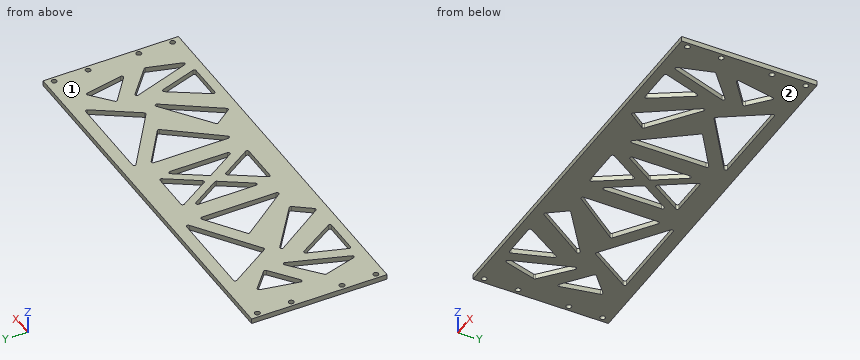
from build123d import *

# Parameters (mm, degrees)
SKETCH_1_W             = 230
SKETCH_1_H             = 80
EXTRUDE_1_DEPTH        = 3
SKETCH_2_R             = 1.55
CUT_EXTRUDE_1_DEPTH    = 3
CUT_EXTRUDE_3_DEPTH    = 3
FILLET_1_R             = 1
CUT_EXTRUDE_4_DEPTH    = 3
FILLET_2_R             = 1
FILLET_2_OF_MIRROR_2_R = 1


with BuildPart() as part:
    # 草图1 → 凸台-拉伸1 (new body)
    with BuildSketch(Plane.XY):
        Rectangle(SKETCH_1_W, SKETCH_1_H)
    extrude(amount=EXTRUDE_1_DEPTH)

    # 草图2 → 切除-拉伸1 (cut)
    with BuildSketch(Plane.XY.offset(3)):
        with Locations((-112, 35)):
            Circle(SKETCH_2_R)
        with Locations((-112, 15)):
            Circle(SKETCH_2_R)
        with Locations((-112, -15)):
            Circle(SKETCH_2_R)
        with Locations((-112, -35)):
            Circle(SKETCH_2_R)
    cut_extrude_1 = extrude(amount=-CUT_EXTRUDE_1_DEPTH, mode=Mode.SUBTRACT)

    # 镜向1: 切除-拉伸1 across plane
    add(cut_extrude_1.mirror(Plane(origin=(0, 0, 0), x_dir=(0, 0, 1), z_dir=(1, 0, 0))), mode=Mode.SUBTRACT)

    # 草图3 → 切除-拉伸3 (cut)
    with BuildSketch(Plane.XY.offset(3)):
        Polygon((-13.305143171, 26.275790798), (13.305143171, 26.275790798), (0, 5.552735947), align=None)
        Polygon((-15.79638841, 21.645852354), (-15.79638841, -19.238624417), (-2.671542174, 1.203613969), align=None)
        Polygon((13.305143171, -26.275790798), (0, -5.552735947), (-13.305143171, -26.275790798), align=None)
        Polygon((15.79638841, -19.238624417), (2.671542174, 1.203613969), (15.79638841, 21.645852354), align=None)
    extrude(amount=-CUT_EXTRUDE_3_DEPTH, mode=Mode.SUBTRACT)

    # 圆角1
    fillet_1_edges = [part.edges().sort_by_distance(p)[0] for p in [
        (13.305143171, -26.275790798, 1.5),
        (-13.305143171, -26.275790798, 1.5),
        (0, -5.552735947, 1.5),
        (-2.671542174, 1.203613969, 1.5),
        (-15.79638841, -19.238624417, 1.5),
        (-15.79638841, 21.645852354, 1.5),
        (15.79638841, 21.645852354, 1.5),
        (15.79638841, -19.238624417, 1.5),
        (2.671542174, 1.203613969, 1.5),
        (13.305143171, 26.275790798, 1.5),
        (0, 5.552735947, 1.5),
        (-13.305143171, 26.275790798, 1.5),
    ]]
    fillet(fillet_1_edges, radius=FILLET_1_R)

    # 草图4 → 切除-拉伸4 (cut)
    with BuildSketch(Plane.XY.offset(3)):
        Polygon((-94.647300932, 26.28167583), (-99.803832265, 0), (-81.173783576, 14.471555678), align=None)
        Polygon((-83.336199942, 32.768924927), (-26.780694991, 32.768924927), (-65.537849854, 5.489210775), align=None)
        Polygon((-79.676726092, 5.489210775), (-99.803832265, -11.810120151), (-93.256525701, -34.501763578), align=None)
        Polygon((-72.690457833, 1.663397204), (-39.739437394, -22.7240812), (-48.404858649, -34.432322132), align=None)
        Polygon((-78.179668608, -9.458541946), (-86.494255189, -34.432322132), (-62.543734886, -34.432322132), align=None)
        Polygon((-50.432218288, 6.882727449), (-26.319327505, 23.854890919), (-26.319327505, -25.008988453), align=None)
    cut_extrude_4 = extrude(amount=-CUT_EXTRUDE_4_DEPTH, mode=Mode.SUBTRACT)

    # 圆角2
    fillet_2_edges = [part.edges().sort_by_distance(p)[0] for p in [
        (-48.404858649, -34.432322132, 1.5),
        (-72.690457833, 1.663397204, 1.5),
        (-39.739437394, -22.7240812, 1.5),
        (-78.179668608, -9.458541946, 1.5),
        (-62.543734886, -34.432322132, 1.5),
        (-86.494255189, -34.432322132, 1.5),
        (-65.537849854, 5.489210775, 1.5),
        (-83.336199942, 32.768924927, 1.5),
        (-26.780694991, 32.768924927, 1.5),
        (-79.676726092, 5.489210775, 1.5),
        (-93.256525701, -34.501763578, 1.5),
        (-99.803832265, -11.810120151, 1.5),
        (-26.319327505, -25.008988453, 1.5),
        (-50.432218288, 6.882727449, 1.5),
        (-26.319327505, 23.854890919, 1.5),
        (-94.647300932, 26.28167583, 1.5),
        (-81.173783576, 14.471555678, 1.5),
        (-99.803832265, 0, 1.5),
    ]]
    fillet(fillet_2_edges, radius=FILLET_2_R)

    # 镜向2: 切除-拉伸4 across plane
    add(cut_extrude_4.mirror(Plane(origin=(0, 0, 0), x_dir=(0, 0, 1), z_dir=(1, 0, 0))), mode=Mode.SUBTRACT)

    # 圆角2 of 镜向2
    fillet_2_of_mirror_2_edges = [part.edges().sort_by_distance(p)[0] for p in [
        (48.404858649, -34.432322132, 1.5),
        (72.690457833, 1.663397204, 1.5),
        (39.739437394, -22.7240812, 1.5),
        (78.179668608, -9.458541946, 1.5),
        (62.543734886, -34.432322132, 1.5),
        (86.494255189, -34.432322132, 1.5),
        (65.537849854, 5.489210775, 1.5),
        (83.336199942, 32.768924927, 1.5),
        (26.780694991, 32.768924927, 1.5),
        (79.676726092, 5.489210775, 1.5),
        (93.256525701, -34.501763578, 1.5),
        (99.803832265, -11.810120151, 1.5),
        (26.319327505, -25.008988453, 1.5),
        (50.432218288, 6.882727449, 1.5),
        (26.319327505, 23.854890919, 1.5),
        (94.647300932, 26.28167583, 1.5),
        (81.173783576, 14.471555678, 1.5),
        (99.803832265, 0, 1.5),
    ]]
    fillet(fillet_2_of_mirror_2_edges, radius=FILLET_2_OF_MIRROR_2_R)


solid = part.part
Check sheet for the modelled part. Datum: model origin and axes. Units: mm. Face numbers are marked on the shaded views. Coordinates: 2 decimals unless noted, no trailing zeros. Loops run counter-clockwise (first coordinate to the right, second up) from the corner with the lowest first, then second, coordinate; pieces in that order, holes last. Notation, with made-up numbers: (63.25, 67) -> (121.25, 67) arc R21 cw to (121.25, 105) -> close; hole circle Ø2 at (82.5, 77.5). An arc over 180 degrees is marked (long way). Write item = value, one per line. Start each with the question number.
1. Material ranges on line 1 (Y direction, x = 112, z = 0.9); line 2 (X direction, y = -34.5, z = 2.8); line 3 (Y direction, x = -66, z = 2), recorded low to high.
2. Section check A-A on x = 73.5. Record the cut outline in (y, z).
3. Depth check by flat-ended pin: P1, Ø1.9, axis at x = -112, y = -35, coming from the +Z side. Enter the tip coordinate at first touch or a pass-through.
4. Draft check along Z on the marked faces 1 and 2. Enter one of: released by +Z, released by -Z, zero draft, split by the parting line, or undercut.
5. Section check B-B on z = 2.35. Give the number of separate pieces and of enclosed holes in the cut face, then the cut area to 3 significant figures.
Responses:
q1.line_1 = -40 to -36.55, -33.45 to -16.55, -13.45 to 13.45, 16.55 to 33.45, 36.55 to 40
q1.line_2 = -115 to -113.47, -110.53 to 110.53, 113.47 to 115
q1.line_3 = -40 to -34.43, -28.91 to -8.28, -3.29 to 6.22, 32.77 to 40
q2.outline = (-40, 0) -> (-34.43, 0) -> (-34.43, 3) -> (-40, 3) -> close; (-16.93, 0) -> (17.69, 0) -> (17.69, 3) -> (-16.93, 3) -> close; (32.77, 0) -> (40, 0) -> (40, 3) -> (32.77, 3) -> close
q3.P1 = through
q4.face_1 = released by +Z
q4.face_2 = released by -Z
q5.separate_pieces = 1
q5.enclosed_holes = 24
q5.area = 12,400 mm2
